Build history of the part. All positions in model axes, mm. Face numbers are marked on the shaded views. A direction names the side the tool comes from. Give positions to 0.01 mm unless a question says otherwise; leave off trailing zeros. Loops run counter-clockwise (first coordinate to the right, second up) from the corner with the lowest first, then second, coordinate; pieces in that order, holes last. Notation, with made-up numbers: M 13,69.5 L 55,69.5 A33 ccw 55,104.5 Z; hole C 30,-7 d10. An arc over 180 degrees is marked long. Put each result on its own line as item: value.
```python
from build123d import *

# Parameters (mm, degrees)
ESQUISSE1_W             = 36
ESQUISSE1_H             = 36
BOSS_EXTRU_1_DEPTH      = 1
D_GAGEMENT_M21_D        = 2.4
ESQUISSE5_W             = 6
ESQUISSE5_H             = 24
ESQUISSE5_W_2           = 24
ESQUISSE5_H_2           = 6
BOSS_EXTRU_2_DEPTH      = 6
BOSS_EXTRU_2_DEPTH_BACK = 7


with BuildPart() as part:
    # Esquisse1 → Boss.-Extru.1 (new body)
    with BuildSketch(Plane(origin=(0, 0, 0), x_dir=(1, 0, 0), z_dir=(0, 1, 0))):
        with Locations((18, 18)):
            Rectangle(ESQUISSE1_W, ESQUISSE1_H)
    extrude(amount=BOSS_EXTRU_1_DEPTH)

    # Dégagement M21 (through all)
    with Locations(Plane(origin=(0, 1, 0), x_dir=(1, 0, 0), z_dir=(0, 1, 0))):
        with Locations((2.75, 2.75), (2.75, 33.25), (33.25, 33.25), (33.25, 2.75)):
            Hole(D_GAGEMENT_M21_D / 2)

    # Esquisse5 → Boss.-Extru.2 (add, two sides)
    with BuildSketch(Plane(origin=(0, 1, 0), x_dir=(1, 0, 0), z_dir=(0, 1, 0))) as boss_extru_2_sk:
        with Locations((3, 18)):
            Rectangle(ESQUISSE5_W, ESQUISSE5_H)
        with Locations((18, 18)):
            Rectangle(ESQUISSE5_W_2, ESQUISSE5_H)
        with Locations((18, 33)):
            Rectangle(ESQUISSE5_W_2, ESQUISSE5_H_2)
        with Locations((33, 18)):
            Rectangle(ESQUISSE5_W, ESQUISSE5_H)
        with Locations((18, 3)):
            Rectangle(ESQUISSE5_W_2, ESQUISSE5_H_2)
    extrude(amount=BOSS_EXTRU_2_DEPTH)
    extrude(boss_extru_2_sk.sketch, amount=-BOSS_EXTRU_2_DEPTH_BACK)


solid = part.part
```
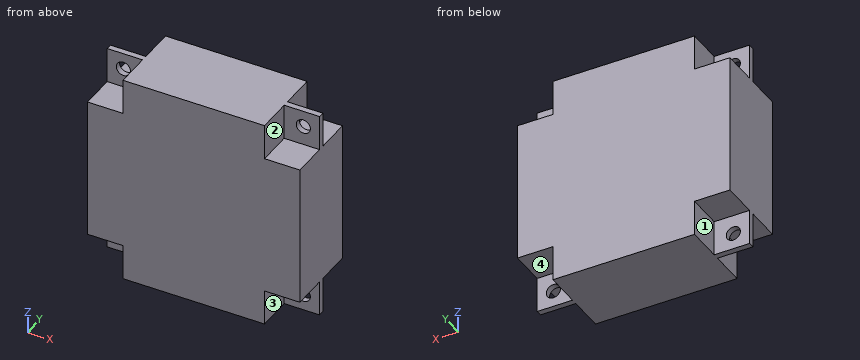
Q1. Drop flat-ended pins along their axis: pin 1 Ø6.5 at (x, y) = (32, -3) entering from -Z; pin 2 Ø1.8 at (x, y) = (1.5, -1.5) entering from -Z; pin 3 Ø1.8 at (x, z) = (33.5, -34) entering from -Y; pin 4 Ø3 at (y, z) = (4, -32) entering from +X. Give the stop position or say it passes through.
Here are the results:
pin 1: z = -36
pin 2: z = -30
pin 3: y = 0
pin 4: x = 30
Q2. Slice it at A-A (x = 2.75). List the corners of the cut face in (y, z).
Here are the results:
outline: M -6,-30 L 0,-30 L 0,-32.05 L 1,-32.05 L 1,-30 L 7,-30 L 7,-6 L 1,-6 L 1,-3.95 L 0,-3.95 L 0,-6 L -6,-6 Z; M 0,-36 L 1,-36 L 1,-34.45 L 0,-34.45 Z; M 0,-1.55 L 1,-1.55 L 1,0 L 0,0 Z
Q3. Tool access for the marked faces 1, 2, 3 and 4: list every direction of +Z, -Z, +X, -X, +Y, -Y with a clear straight run to the whole face (end or side of a thin tool).
Here are the results:
face 1: -Z, -X, +Y
face 2: +Z, +X, -Y
face 3: -Z, +X, -Y
face 4: -Z, +X, +Y
Q4. Slice it at D-D (y = -3.25). List the corners of the cut face in (x, z).
Here are the results:
outline: M 0,-30 L 6,-30 L 6,-36 L 30,-36 L 30,-30 L 36,-30 L 36,-6 L 30,-6 L 30,0 L 6,0 L 6,-6 L 0,-6 Z
Q5. Probe line 1 (X direction, y = 0.3, z = -33.25); line 2 (Z direction, x = 2.75, y = 0.65); line 3 (X direction, y = 5.25, z = -32.5). List the from-to ranges inside material, lowest first. Write a range as from..to.
Here are the results:
line 1: 0..1.55, 3.95..32.05, 34.45..36
line 2: -36..-34.45, -32.05..-3.95, -1.55..0
line 3: 6..30
Q6. Slice it at B-B (z = -2.75). List the corners of the cut face in (x, y), and give its area (3 significant figures).
Here are the results:
outline: M 0,0 L 1.55,0 L 1.55,1 L 0,1 Z; M 3.95,0 L 6,0 L 6,-6 L 30,-6 L 30,0 L 32.05,0 L 32.05,1 L 30,1 L 30,7 L 6,7 L 6,1 L 3.95,1 Z; M 34.45,0 L 36,0 L 36,1 L 34.45,1 Z
area: 319 mm²
Q7. Slice it at C-C (z = -31). List the corners of the cut face in (x, y).
Here are the results:
outline: M 0,0 L 6,0 L 6,-6 L 30,-6 L 30,0 L 36,0 L 36,1 L 30,1 L 30,7 L 6,7 L 6,1 L 0,1 Z
